```python
from build123d import *

# Parameters (mm, degrees)
SKETCH1_W                                       = 278
SKETCH1_H                                       = 278
BOSS_EXTRUDE1_DEPTH                             = 6.35
CHAMFER1_SIZE                                   = 20
SKETCH4_R                                       = 2.75
CUT_EXTRUDE2_DEPTH                              = 76.2
SKETCH8_R                                       = 17.5
CUT_EXTRUDE4_DEPTH                              = 105
CSK_FOR_M4_FLAT_HEAD_MACHINE_SCREW2_D           = 4.5
CSK_FOR_M4_FLAT_HEAD_MACHINE_SCREW2_CSINK_D     = 9.4
CSK_FOR_M4_FLAT_HEAD_MACHINE_SCREW2_CSINK_ANGLE = 90
CSK_FOR_M3_FLAT_HEAD_MACHINE_SCREW1_D           = 3.4
CSK_FOR_M3_FLAT_HEAD_MACHINE_SCREW1_CSINK_D     = 6.3
CSK_FOR_M3_FLAT_HEAD_MACHINE_SCREW1_CSINK_ANGLE = 90
CSK_FOR_M3_FLAT_HEAD_MACHINE_SCREW2_D           = 3.4
CSK_FOR_M3_FLAT_HEAD_MACHINE_SCREW2_CSINK_D     = 6.3
CSK_FOR_M3_FLAT_HEAD_MACHINE_SCREW2_CSINK_ANGLE = 90


with BuildPart() as part:
    # Sketch1 → Boss-Extrude1 (new body)
    with BuildSketch(Plane.XY):
        Rectangle(SKETCH1_W, SKETCH1_H)
    extrude(amount=BOSS_EXTRUDE1_DEPTH)

    # Chamfer1
    chamfer1_edges = [part.edges().sort_by_distance(p)[0] for p in [
        (-139, 139, 3.175),
        (139, 139, 3.175),
        (139, -139, 3.175),
        (-139, -139, 3.175),
    ]]
    chamfer(chamfer1_edges, length=CHAMFER1_SIZE)

    # Sketch4 → Cut-Extrude2 (cut)
    with BuildSketch(Plane.XY.offset(6.35)):
        with Locations((-90, 130)):
            Circle(SKETCH4_R)
        with Locations((0, 130)):
            Circle(SKETCH4_R)
        with Locations((90, 130)):
            Circle(SKETCH4_R)
        with Locations((90, -130)):
            Circle(SKETCH4_R)
        with Locations((0, -130)):
            Circle(SKETCH4_R)
        with Locations((-90, -130)):
            Circle(SKETCH4_R)
    extrude(amount=-CUT_EXTRUDE2_DEPTH, mode=Mode.SUBTRACT)

    # Sketch8 → Cut-Extrude4 (cut)
    with BuildSketch(Plane.XY.offset(6.35)):
        with Locations((0, 79)):
            Circle(SKETCH8_R)
        with Locations((0, -79)):
            Circle(SKETCH8_R)
    extrude(amount=-CUT_EXTRUDE4_DEPTH, mode=Mode.SUBTRACT)

    # CSK for M4 Flat Head Machine Screw2 (through all)
    with Locations(Plane.XY.offset(6.35)):
        with Locations((27.5, 79), (-27.5, 79), (-27.5, -79), (27.5, -79)):
            CounterSinkHole(CSK_FOR_M4_FLAT_HEAD_MACHINE_SCREW2_D / 2, CSK_FOR_M4_FLAT_HEAD_MACHINE_SCREW2_CSINK_D / 2, counter_sink_angle=CSK_FOR_M4_FLAT_HEAD_MACHINE_SCREW2_CSINK_ANGLE)

    # CSK for M3 Flat Head Machine Screw1 (through all)
    with Locations(Plane.XY.offset(6.35)):
        with Locations((-131, 30), (-120, 30), (-120, -30), (-131, -30), (131, -30), (120, -30), (120, 30), (131, 30)):
            CounterSinkHole(CSK_FOR_M3_FLAT_HEAD_MACHINE_SCREW1_D / 2, CSK_FOR_M3_FLAT_HEAD_MACHINE_SCREW1_CSINK_D / 2, counter_sink_angle=CSK_FOR_M3_FLAT_HEAD_MACHINE_SCREW1_CSINK_ANGLE)

    # CSK for M3 Flat Head Machine Screw2 (through all)
    with Locations(Plane.XY.offset(6.35)):
        with Locations((-45.858494434, 36.37268476), (-53.858494434, -39.12731524), (36.641505566, 40.37268476), (49.141505566, -39.12731524)):
            CounterSinkHole(CSK_FOR_M3_FLAT_HEAD_MACHINE_SCREW2_D / 2, CSK_FOR_M3_FLAT_HEAD_MACHINE_SCREW2_CSINK_D / 2, counter_sink_angle=CSK_FOR_M3_FLAT_HEAD_MACHINE_SCREW2_CSINK_ANGLE)


solid = part.part
```
Input: part model. Units: mm. Frame: model coordinates. Coordinates: 2 decimals unless noted, no trailing zeros. Answer as a JSON object with one key per item and string values.
1. Material intervals for line 1 (Y direction, x = 0, z = 4); line 2 (X direction, y = -39, z = 3.75); line 3 (Y direction, x = -27.5, z = 2.45), sorted ascending. Write a range as from..to.
Result set:
{"line 1": "y = -139..-132.75, -127.25..-96.5, -61.5..61.5, 96.5..127.25, 132.75..139", "line 2": "x = -139..-55.55, -52.16..47.45, 50.84..139", "line 3": "y = -139..-81.25, -76.75..76.75, 81.25..139"}
2. Mould query, pull axis Y, two halves, no side actions, for faces 1 (the face through (-129, 129, 3)), 2 (the face through (-2, 2, 6.35)), 3 (the face through (-3.794, -96.084, 3.219)). Classes: released by +Y, released by -Y, zero draft, split by the parting line, or undercut.
Result set:
{"face 1": "released by +Y", "face 2": "zero draft", "face 3": "undercut"}
3. First-contact query: P1, Ø7, axis at x = 27.5, y = 79, coming from the +Z side; P2, Ø5, axis at x = -27.5, y = 79, coming from the +Z side; P3, Ø5.5, axis at x = -45.86, y = 36.37, coming from the +Z side; P4, Ø3.5, axis at x = 90, y = 130, coming from the -Z side. Flat tips, straight axial feed; report the tip coordinate or a pass-through.
Result set:
{"P1": "stops at z = 5.15", "P2": "stops at z = 4.15", "P3": "stops at z = 5.95", "P4": "passes through"}
4. Section A-A on z = 2. Count the separate pieces of the cut face and the enclosed holes in it, then the cut area to 3 significant figures.
Result set:
{"separate pieces": "1", "enclosed holes": "24", "area": "74,200 mm2"}
